from build123d import *

# Parameters (mm, degrees)
F0_W     = 79.502
F0_H     = 44.196
F1_DEPTH = 40.64
F3_T     = -14.732
F4_D     = 13.97
F6_W     = 20.32
F6_H     = 44.196
F7_DEPTH = 40.64
F8_D     = 13.97
F9_R     = 22.09799
F10_R    = 20.31999


# Not quite as in the source:
# - a fillet or chamfer is up to 0.001 mm smaller than in the source, because OpenCascade refuses the exact size


with BuildPart() as f1:
    # F0 (on Right) → F1 (new body)
    with BuildSketch(Plane.YZ):
        with Locations((39.751, 22.098)):
            Rectangle(F0_W, F0_H)
    extrude(amount=F1_DEPTH)

    # F3
    f3_openings = [f1.faces().sort_by_distance(p)[0] for p in [
        (40.64, 39.751, 22.098),
        (20.32, 79.502, 22.098),
        (0, 39.751, 22.098),
    ]]
    offset(amount=F3_T, openings=f3_openings)

    # F4 (through all)
    with Locations(Plane.XY.offset(44.196)):
        with Locations((20.32, 59.182)):
            Hole(F4_D / 2)

    # F6 (on face) → F7 (join)
    with BuildSketch(Plane(origin=(0, 0, 0), x_dir=(0, -1, 0), z_dir=(-1, 0, 0))):
        with Locations((10.16, 22.098)):
            Rectangle(F6_W, F6_H)
    extrude(amount=-F7_DEPTH)

    # F8 (through all)
    with Locations(Plane.YZ.offset(40.64)):
        with Locations((-9.398, 22.098)):
            Hole(F8_D / 2)

    # F9 (radius 22.098 in the source; OpenCascade refuses exactly that, so slightly less here)
    f9_edges = [f1.edges().sort_by_distance(p)[0] for p in [
        (20.32, -20.32, 44.196),
        (20.32, -20.32, 0),
    ]]
    fillet(f9_edges, radius=F9_R)

    # F10 (radius 20.32 in the source; OpenCascade refuses exactly that, so slightly less here)
    f10_edges = [f1.edges().sort_by_distance(p)[0] for p in [
        (0, 79.502, 36.83),
        (0, 79.502, 7.366),
        (40.64, 79.502, 7.366),
        (40.64, 79.502, 36.83),
    ]]
    fillet(f10_edges, radius=F10_R)


solid = f1.part
Model file for the job. Use its own axes, mm. A direction names the side the tool comes from. Give positions to 0.01 mm unless a question says otherwise; leave off trailing zeros. Loops run counter-clockwise (first coordinate to the right, second up) from the corner with the lowest first, then second, coordinate; pieces in that order, holes last.
1) Saw through at B-B (x = 16). Count the separate pieces of the cut face and the enclosed holes in it, plus the area to 3 significant figures.
2) Wall check: line 1 (Z direction, x = 13, y = 34); line 2 (Y direction, x = 11, z = 18.5); line 3 (Y direction, x = 20.32, z = 10.5). Give the ranges that are in metal, low to high.
3) Saw through at C-C (z = 25). Write the cut outline in (x, y).
4) Tool access for faces 5 (the cylindrical face through (5.8, 73.4, 7.5)), 6 (the flat face through (20, 47, 29.464)): list every direction of +Z, -Z, +X, -X, +Y, -Y with a clear straight run to the whole face (end or side of a thin tool).
5) Saw through at A-A (y = 40). Write the cut outline in (x, z).
6) Pull direction Z, two halves, no side cores. Call faces 1 (the flat face through (20, 41, 0)), 2 (the cylindrical face through (17.097, 52.985, 36.727)), 3 (the flat face through (20, 14.732, 22)), 4 (the flat face through (20, 47, 14.732)): +Z half, -Z half, draft (parallel to the pull), parting line (faces both ways), or undercut.
7) Flat gauge pins, fed straight in: pin 1 Ø16 at (x, z) = (11, 22.5) entering from +Y; pin 2 Ø6 at (x, z) = (14.5, 26) entering from +Y; pin 3 Ø8.5 at (y, z) = (-9.398, 22.098) entering from -X. Where does each tip first touch, or does it go through?
Answer block:
1. separate pieces: 3
1. enclosed holes: 1
1. area: 2,760 mm2
2. line 1: z = 0 to 14.73, 29.46 to 44.2
2. line 2: y = -20.03 to -15.39, -3.41 to 14.73
2. line 3: y = -17.03 to 52.2, 66.17 to 79.5
3. outline: (0, -20.13) - (40.64, -20.13) - (40.64, -15.75) - (0, -15.75) - close; (0, -3.04) - (40.64, -3.04) - (40.64, 14.73) - (0, 14.73) - close
4. face 5: +Z, -Z, -X, +Y
4. face 6: +X, -X, +Y
5. outline: (0, 0) - (40.64, 0) - (40.64, 14.73) - (0, 14.73) - close; (0, 29.46) - (40.64, 29.46) - (40.64, 44.2) - (0, 44.2) - close
6. face 1: -Z half
6. face 2: draft
6. face 3: undercut
6. face 4: undercut
7. pin 1: stops at y = 78.78
7. pin 2: stops at y = 14.73
7. pin 3: passes through
